from build123d import *

# Parameters (mm, degrees)
F0_R     = 15.875
F0_R_2   = 14.2875
F1_DEPTH = 9.525
F2_W     = 38.1
F2_H     = 50.8
F2_R     = 14.2875
F3_DEPTH = 4.7625
F4_W     = 38.1
F4_H     = 50.8
F4_W_2   = 31.75
F4_H_2   = 44.45
F5_DEPTH = 177.8


with BuildPart() as f1:
    # F0 (on Front) → F1 (new body)
    with BuildSketch(Plane.XZ):
        Circle(F0_R)
        Circle(F0_R_2, mode=Mode.SUBTRACT)
    extrude(amount=F1_DEPTH)

    # F2 (on Front) → F3 (join)
    with BuildSketch(Plane.XZ):
        with Locations((0, -6.35)):
            Rectangle(F2_W, F2_H)
        Circle(F2_R, mode=Mode.SUBTRACT)
    extrude(amount=-F3_DEPTH)

    # F4 (on face) → F5 (join)
    with BuildSketch(Plane(origin=(0, 4.7625, 0), x_dir=(-1, 0, 0), z_dir=(0, 1, 0))):
        with Locations((0, -6.35)):
            Rectangle(F4_W, F4_H)
        with Locations((0, -6.35)):
            Rectangle(F4_W_2, F4_H_2, mode=Mode.SUBTRACT)
    extrude(amount=F5_DEPTH)


solid = f1.part
Part model, mm, in its own coordinate system. A direction names the side the tool comes from. Coordinates: 2 decimals unless noted, no trailing zeros. Write each loop counter-clockwise with the first axis right and the second up, starting at its lowest first coordinate (ties: lowest second). Pieces come first, ordered by that corner, then holes. Notation, with made-up numbers: M 8,-39.75 L 41,-39.75 A26 cw 41,-23.75 Z; hole C 63,36.5 d7. An arc over 180 degrees is marked long. Return JSON: item names as keys, results as strings.
1. Saw through at B-B, the plane y = 122.5. Write the cut outline in (x, z) (3 decimals), then the cut area to 3 significant figures.
Determined:
{"outline": "M -19.05,-31.75 L 19.05,-31.75 L 19.05,19.05 L -19.05,19.05 Z; hole M -15.875,-28.575 L 15.875,-28.575 L 15.875,15.875 L -15.875,15.875 Z", "area": "524 mm²"}
2. Pull direction Z, two halves, no side cores. Call faces 4 (the face through (-3.441, -4.696, -15.497)), 5 (the face through (0, 90, 19.05)), 6 (the face through (15.875, 92, -7)), 7 (the face through (0, 92, -28.575)): pulls with the +Z half, pulls with the -Z half, needs draft (parallel to the pull), parting line crosses it, or undercut.
Determined:
{"face 4": "parting line crosses it", "face 5": "pulls with the +Z half", "face 6": "undercut", "face 7": "undercut"}
3. 3-axis set-ups, long thin cutter, end or side, ignore diameter. For faces 1 (the face through (0, 0, -17)), 2 (the face through (-15.875, 92, -7)), 3 (the face through (-19.05, 90, -7)): which of +Z, -Z, +X, -X, +Y, -Y reach the whole face in a straight line?
Determined:
{"face 1": "-Y", "face 2": "+Y", "face 3": "+Z, -Z, -X, +Y, -Y"}
4. Probe L1, parallel to Z at x = 11.5, y = 46.5 (3 decimals); L2, parallel to X at y = 45, z = 5.5 (3 decimals); L3, parallel to Z at x = 0, y = -2.75 (1 decimal). List the from-to ranges inside material, lowest first.
Determined:
{"L1": "-31.75 to -28.575, 15.875 to 19.05", "L2": "-19.05 to -15.875, 15.875 to 19.05", "L3": "-15.9 to -14.3, 14.3 to 15.9"}
5. Flat gauge pins, fed straight in: pin 1 Ø6 at (x, z) = (12, 9) entering from +Y; pin 2 Ø12 at (x, z) = (8, -22) entering from -Y. Where does each tip first touch, or does it go through?
Determined:
{"pin 1": "y = 4.76", "pin 2": "y = 0"}
